Drawing for the job (mm, zero at the part's lowest x, y, z). A direction names the side the tool comes from. Round coordinates to 2 decimals unless told otherwise and drop trailing zeros. Answer in a Markdown table with one row per item.
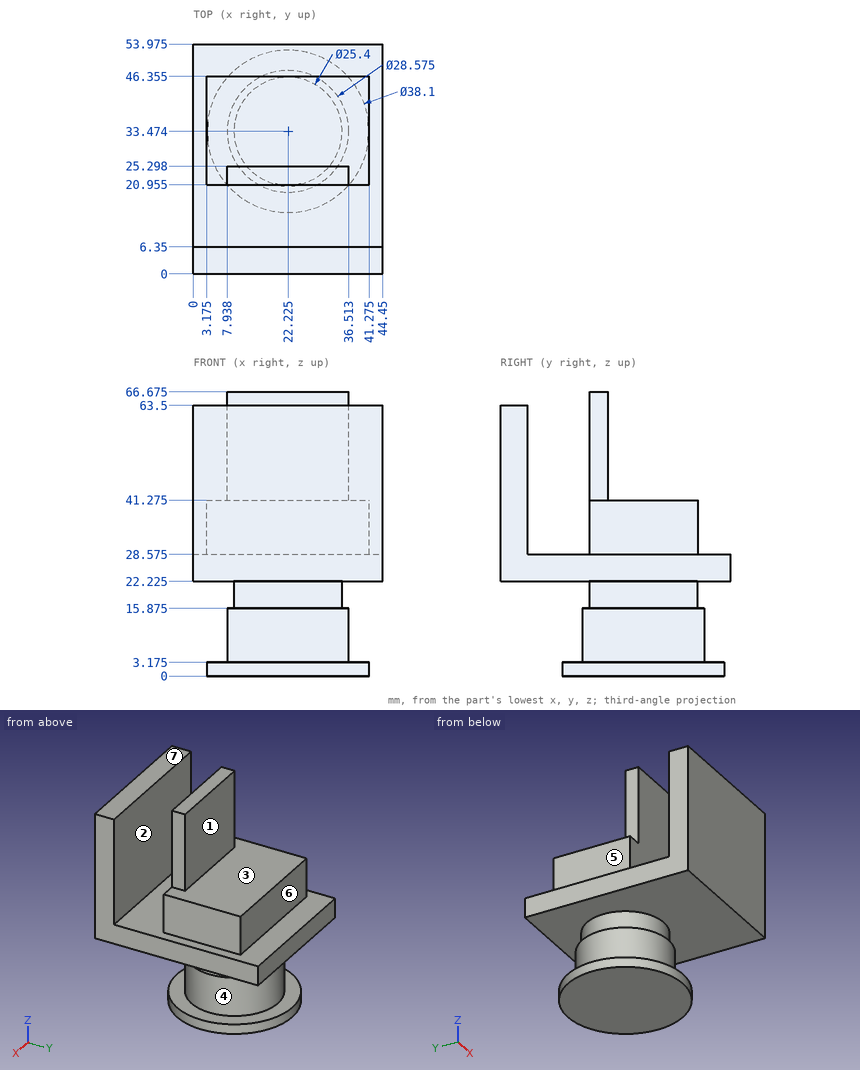
1. Wall check: probe 1 along Z at (x, y) = (9, 25.5) (1 decimal); probe 2 along Z at (x, y) = (32, 22.5) (1 decimal); probe 3 along Y at (x, z) = (3, 38). Give the ranges that are in metal, low to high.
Verdict:
| item | result |
|---|---|
| probe 1 | z = 0 to 3.2, 22.2 to 41.3 |
| probe 2 | z = 0 to 3.2, 22.2 to 66.7 |
| probe 3 | y = 0 to 6.35 |
2. Pin check, flat tips, straight feed: pin 1 (17.5 mm diameter, centred on x = 23.5, z = 52, fed in from +Y); pin 2 (10 mm diameter, centred on x = 13.5, y = 41.5, fed in from -Z); pin 3 (1.9 mm diameter, centred on x = 12, y = 4, fed in from +Z); pin 4 (4 mm diameter, centred on y = 28.5, z = 33, fed in from +X) (1 decimal). Stop position of each tip, or through.
Verdict:
| item | result |
|---|---|
| pin 1 | stops at y = 25.3 |
| pin 2 | stops at z = 0 |
| pin 3 | stops at z = 63.5 |
| pin 4 | stops at x = 41.3 |
3. Mould opens along Y. For the marked faces 1, 2 and 3 say: +Y half, -Y half, draft (parallel to the pull), parting line (faces both ways), or undercut.
Verdict:
| item | result |
|---|---|
| face 1 | +Y half |
| face 2 | undercut |
| face 3 | draft |
4. Tool access for the marked faces 4, 5, 6 and 7: list every direction of +Z, -Z, +X, -X, +Y, -Y with a clear straight run to the whole face (end or side of a thin tool).
Verdict:
| item | result |
|---|---|
| face 4 | none |
| face 5 | +Z, -X, +Y |
| face 6 | +Z, +X, -X, +Y |
| face 7 | +Z, +X, -X, -Y |
